Here's how the part is built. I have some questions about the finished solid (model axes, mm). Round coordinates to 2 decimals unless told otherwise and drop trailing zeros. Loops run counter-clockwise (first coordinate to the right, second up) from the corner with the lowest first, then second, coordinate; pieces in that order, holes last. Notation, with made-up numbers: M 37,-39 L 53,-39 A8 cw 53,-32 Z; hole C 14.25,51.25 d7. An arc over 180 degrees is marked long. One line per question, with ' | ' between items. Start each with the question number.
```python
from build123d import *

# Parameters (mm, degrees)
CYLINDER416_R     = 5
CYLINDER416_DEPTH = 4
CYLINDER415_R     = 7.5
CYLINDER415_DEPTH = 4


with BuildPart() as cylinder:
    # Cylinder416 → Cylinder416 (new body)
    with BuildSketch(Plane(origin=(75, 69, 46), x_dir=(1, 0, 0), z_dir=(0, -1, 0))):
        Circle(CYLINDER416_R)
    extrude(amount=CYLINDER416_DEPTH)


with BuildPart() as cut004026018020025012002:
    # Cylinder415 → Cylinder415 (new body)
    with BuildSketch(Plane(origin=(75, 69, 46), x_dir=(1, 0, 0), z_dir=(0, -1, 0))):
        Circle(CYLINDER415_R)
    extrude(amount=CYLINDER415_DEPTH)

    # Cut004026018020025012002: cut Cylinder
    add(cylinder.part, mode=Mode.SUBTRACT)


solid = cut004026018020025012002.part
```
1) Imagine slicing it at D-D (z = 40). Write out the boundary of the cut face in (x, y).
2) We'd pull the mould along X, two halves only. Please class faces 1 (the face through (77, 69, 41)), 2 (the face through (78, 67, 50)), 3 (the face through (73.37, 67.03, 38.68)): pulls with the +X half, pulls with the -X half, needs draft (parallel to the pull), parting line crosses it, or undercut.
3) I'm going to push flat-ended pins straight in: pin 1 Ø1.5 at (y, z) = (66.5, 51.5) entering from -X; pin 2 Ø6 at (x, z) = (75, 46) entering from +Y. Where does each tip first touch, or does it pass through?
4) Imagine slicing it at C-C (y = 68.45). Write out the boundary of the cut face in (x, z).
5) Imagine slicing it at B-B (x = 75). Write out the boundary of the cut face in (y, z), then the cut area to 3 significant figures.
6) Please list where these lines run through material, in increasing order: L1, parallel to Z at x = 75, y = 67.8; L2, parallel to Z at x = 73.25, y = 65.8; L3, parallel to X at y = 65.55, z = 46.75. Write a range as from..to.
7) Imagine slicing it at A-A (z = 46). Write out the boundary of the cut face in (x, y), then the cut area to 3 significant figures.
Results are:
1) outline: M 70.5,65 L 79.5,65 L 79.5,69 L 70.5,69 Z
2) face 1: needs draft | face 2: undercut | face 3: parting line crosses it
3) pin 1: x = 69.2 | pin 2: through
4) outline: C 75,46 d15; hole C 75,46 d10
5) outline: M 65,38.5 L 69,38.5 L 69,41 L 65,41 Z; M 65,51 L 69,51 L 69,53.5 L 65,53.5 Z | area: 20.0 mm²
6) L1: 38.5..41, 51..53.5 | L2: 38.71..41.32, 50.68..53.29 | L3: 67.54..70.06, 79.94..82.46
7) outline: M 67.5,65 L 70,65 L 70,69 L 67.5,69 Z; M 80,65 L 82.5,65 L 82.5,69 L 80,69 Z | area: 20.0 mm²
